Print and shaded views of the part. All mm, measured from the part's lowest x, y and z. Round coordinates to 2 decimals unless told otherwise and drop trailing zeros. Order: outer loops, then holes, each group sorted by start corner. A loop starts at its lowest first (then second) coordinate and runs counter-clockwise, first axis right, second up. Notation, with made-up numbers: (75, 9) - (104, 9) arc R10 ccw to (104, 17) - close; hole circle Ø7 at (17, 87.5). An arc over 180 degrees is marked (long way). Write item = value, one per line.
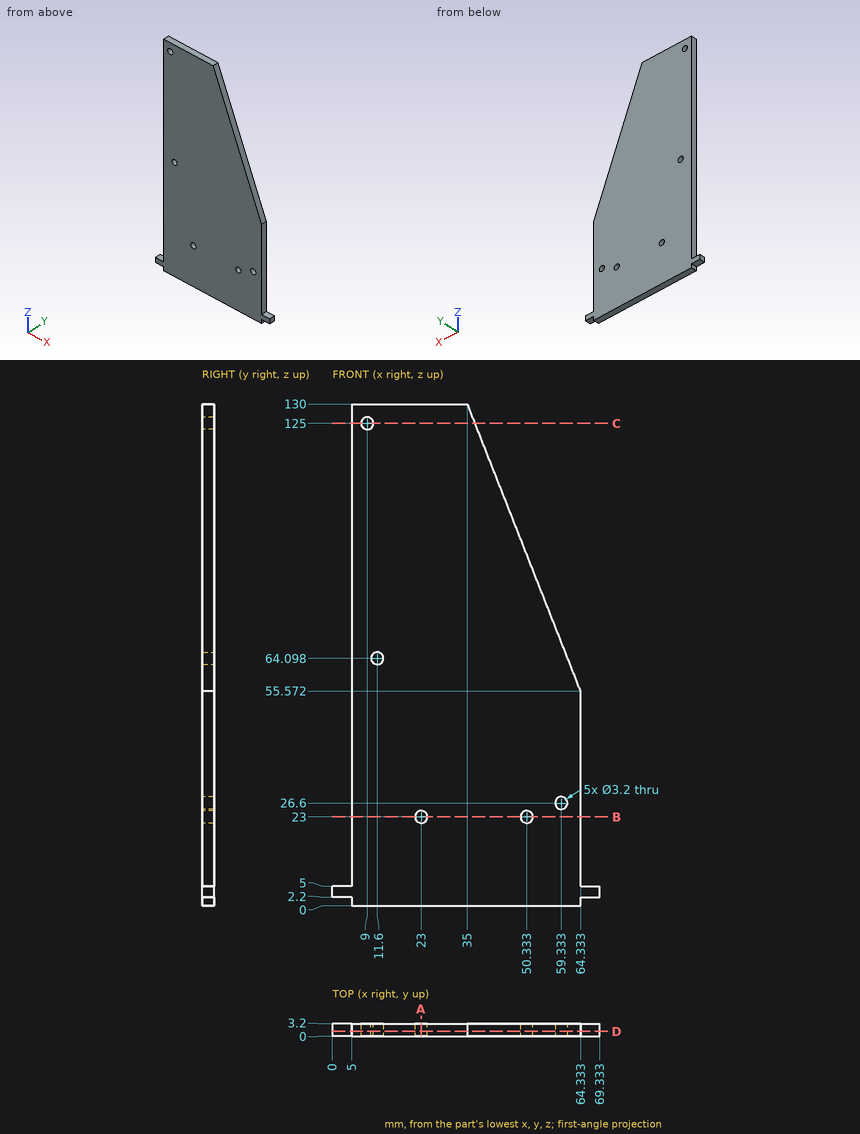
(1) Probe line 1 along Z through (x, y) = (9, 0.9); line 2 along X through (y, z) = (1.5, 39.5); line 3 along X through (y, z) = (2.65, 87). List the from-to ranges inside material, lowest first.
Solved:
line_1 = 0 to 123.4, 126.6 to 130
line_2 = 5 to 64.33
line_3 = 5 to 51.95
(2) Band-saw the part on A-A on x = 23. List the corners of the cut face in (y, z), plus the area to 3 significant figures.
Solved:
outline = (0, 0) - (3.2, 0) - (3.2, 21.4) - (0, 21.4) - close; (0, 24.6) - (3.2, 24.6) - (3.2, 130) - (0, 130) - close
area = 406 mm²
(3) Drop flat-ended pins along their axis: pin 1 (1.8 mm diameter, centred on y = 2, z = 1, fed in from +X); pin 2 (1 mm diameter, centred on x = 3, y = 1.5, fed in from +Z); pin 3 (1 mm diameter, centred on x = 67.5, y = 1, fed in from -Z). Give the stop position or say it passes through.
Solved:
pin_1 = 64.33
pin_2 = 5
pin_3 = 2.2
(4) Band-saw the part on C-C on z = 125. List the corners of the cut face in (x, y).
Solved:
outline = (5, 0) - (7.4, 0) - (7.4, 3.2) - (5, 3.2) - close; (10.6, 0) - (36.97, 0) - (36.97, 3.2) - (10.6, 3.2) - close
(5) Band-saw the part on B-B on z = 23. List the corners of the cut face in (x, y), plus the area to 3 significant figures.
Solved:
outline = (5, 0) - (21.4, 0) - (21.4, 3.2) - (5, 3.2) - close; (24.6, 0) - (48.73, 0) - (48.73, 3.2) - (24.6, 3.2) - close; (51.93, 0) - (64.33, 0) - (64.33, 3.2) - (51.93, 3.2) - close
area = 169 mm²
(6) Band-saw the part on D-D on y = 1.2. List the corners of the cut face in (x, z).
Solved:
outline = (0, 2.2) - (5, 2.2) - (5, 0) - (64.33, 0) - (64.33, 2.2) - (69.33, 2.2) - (69.33, 5) - (64.33, 5) - (64.33, 55.57) - (35, 130) - (5, 130) - (5, 5) - (0, 5) - close; hole circle Ø3.2 at (9, 125); hole circle Ø3.2 at (11.6, 64.1); hole circle Ø3.2 at (23, 23); hole circle Ø3.2 at (50.33, 23); hole circle Ø3.2 at (59.33, 26.6)
